```python
from build123d import *

# Parameters (mm, degrees)
F0_W     = 130.488038063
F0_H     = 78.0766904354
F1_DEPTH = 25
F3_D     = 12.7
F3_DEPTH = 12
F3_TIP   = 3.8154649308


# Not quite as in the source:
# - a length typed as a fraction of an inch, garbled in the dataset ("3 / 203.2 mm" for 3/8 in), is restored


with BuildPart() as f1:
    # F0 (on Front) → F1 (new body)
    with BuildSketch(Plane.XZ):
        with Locations((4.5927464962, -2.1641068161)):
            Rectangle(F0_W, F0_H)
    extrude(amount=F1_DEPTH)

    # F3
    with Locations(Plane(origin=(0, 0, 0), x_dir=(1, 0, 0), z_dir=(0, 1, 0))):
        with Locations((-13.1143694744, 18.479084596), (-5.4509616457, -20.7668524235), (49.2379032075, 5.5906269699)):
            Hole(F3_D / 2, depth=F3_DEPTH)
            with Locations((0, 0, -(F3_DEPTH + F3_TIP / 2))):  # 118° drill point
                Cone(0, F3_D / 2, F3_TIP, mode=Mode.SUBTRACT)


solid = f1.part
```
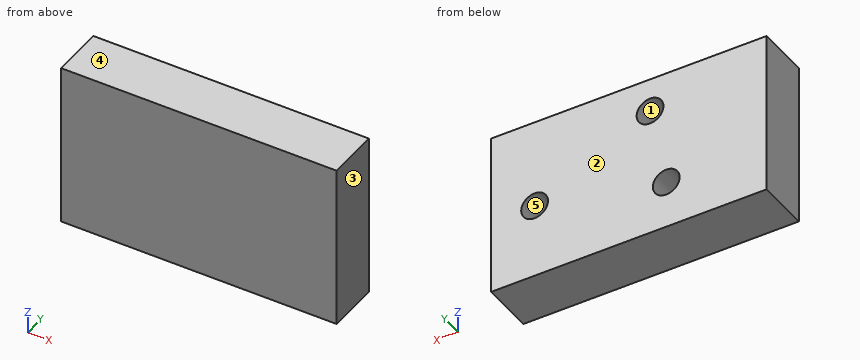
CAD build for the part. Positions are in the model's coordinates, mm. Face numbers are marked on the shaded views. A direction names the side the tool comes from. Round coordinates to 2 decimals unless told otherwise and drop trailing zeros. Order: outer loops, then holes, each group sorted by start corner. A loop starts at its lowest first (then second) coordinate and runs counter-clockwise, first axis right, second up.
Q1. Slice it at A-A (y = -7.5). Write the cut outline in (x, z).
Q2. Wall check: L1, parallel to Z at x = -12.5, y = -2.75; L2, parallel to X at y = -7.5, z = 23; L3, parallel to X at y = -6.5, z = -16. Give the ranges that are in metal, low to high.
Q3. Two-plate mould, pull along X, no slides. Class the marked faces 3, 4 and 5: pulls with the +X half, pulls with the -X half, needs draft (parallel to the pull), parting line crosses it, or undercut.
Q4. Which spindle directions (+Z, -Z, +X, -X, +Y, -Y) get a long thin tool onto all of the face, cutting with end or side? Do the marked faces 1 and 2. Say none if no direction does.
Q5. Drop a flat-ended pin along its axis: pin 1 (11.5 mm diameter, centred on x = -13.11, z = -18.48, fed in from +Y). Give the stop position or say it passes through.
Results below:
1. outline: (-60.65, -41.2) - (69.84, -41.2) - (69.84, 36.87) - (-60.65, 36.87) - close; hole circle Ø12.7 at (-13.11, -18.48); hole circle Ø12.7 at (-5.45, 20.77); hole circle Ø12.7 at (49.24, -5.59)
2. L1: z = -41.2 to -24.8, -12.16 to 36.87
2. L2: x = -60.65 to -11.4, 0.49 to 69.84
2. L3: x = -60.65 to -18.96, -7.27 to 69.84
3. face 3: pulls with the +X half
3. face 4: needs draft
3. face 5: undercut
4. face 1: +Y
4. face 2: +Z, -Z, +X, -X, +Y
5. pin 1: stops at y = -12.36
